```python
from build123d import *

# Parameters (mm, degrees)
BOSS_EXTRUDE1_DEPTH = 152.4
CUT_EXTRUDE1_DEPTH  = 1888.307171607
FILLET1_R           = 10
BOSS_EXTRUDE2_DEPTH = 476.835088
CUT_EXTRUDE2_REACH  = 1889.307
SKETCH4_W           = 50.8
SKETCH4_H           = 222.835087774
SKETCH6_R           = 15.875
CUT_EXTRUDE3_DEPTH  = 1677.259068793
SKETCH7_W           = 40
SKETCH7_H           = 102.835087774
SKETCH7_R           = 5
BOSS_EXTRUDE3_DEPTH = 25.4


with BuildPart() as part:
    # Sketch1 → Boss-Extrude1 (new body)
    with BuildSketch(Plane.XY):
        Polygon((0, 0), (-762, 0), (-1066.8, 304.8), (-1066.8, 787.4), (-812.8, 1549.4), (0, 1549.4), align=None)
    extrude(amount=BOSS_EXTRUDE1_DEPTH)

    # Sketch2 → Cut-Extrude1 (cut, through all)
    with BuildSketch(Plane.XY.offset(152.4)):
        Polygon((-924.463579053, 812.8), (-127, 939.8), (-127, 1435.1), (-717.03024572, 1435.1), align=None)
    extrude(amount=-CUT_EXTRUDE1_DEPTH, mode=Mode.SUBTRACT)

    # Fillet1
    fillet1_edges = [part.edges().sort_by_distance(p)[0] for p in [
        (0, 0, 76.2),
        (-762, 0, 76.2),
        (-1066.8, 304.8, 76.2),
        (-1066.8, 787.4, 76.2),
        (-812.8, 1549.4, 76.2),
        (0, 1549.4, 76.2),
        (-939.8, 1168.4, 152.4),
        (-1066.8, 546.1, 152.4),
        (-914.4, 152.4, 152.4),
        (-820.746912386, 1123.95, 0),
        (-924.463579053, 812.8, 76.2),
        (-422.01512286, 1435.1, 0),
        (-717.03024572, 1435.1, 76.2),
        (-127, 1187.45, 0),
        (-381, 0, 152.4),
        (-127, 1435.1, 76.2),
        (-525.731789526, 876.3, 0),
        (-127, 939.8, 76.2),
        (-820.746912386, 1123.95, 152.4),
        (-525.731789526, 876.3, 152.4),
        (-127, 1187.45, 152.4),
        (-422.01512286, 1435.1, 152.4),
        (0, 774.7, 152.4),
        (-381, 0, 0),
        (-914.4, 152.4, 0),
        (-1066.8, 546.1, 0),
        (-939.8, 1168.4, 0),
        (-406.4, 1549.4, 0),
        (0, 774.7, 0),
        (-406.4, 1549.4, 152.4),
    ]]
    fillet(fillet1_edges, radius=FILLET1_R)

    # Sketch3 → Boss-Extrude2 (add)
    with BuildSketch(Plane(origin=(0, 308.942135624, 0), x_dir=(-1, 0, 0), z_dir=(0, -1, 0))):
        with BuildLine():
            Line((1066.286832981, -76.2), (1066.286832981, -50.8))
            Line((1066.286832981, -50.8), (1091.686832981, -50.8))
            ThreePointArc((1091.686832981, -50.8), (1117.086832981, -76.2), (1091.686832981, -101.6))
            Line((1091.686832981, -101.6), (1066.286832981, -101.6))
            Line((1066.286832981, -101.6), (1066.286832981, -76.2))
        make_face()
    extrude(amount=-BOSS_EXTRUDE2_DEPTH)

    # Sketch4 → Cut-Extrude2 (cut, up to next)
    with BuildSketch(Plane.ZY.offset(1066.8), mode=Mode.PRIVATE) as cut_extrude2_sk1:
        with Locations((76.2, 547.359679511)):
            Rectangle(SKETCH4_W, SKETCH4_H)
    cut_extrude2_tool1 = extrude(cut_extrude2_sk1.sketch, amount=CUT_EXTRUDE2_REACH, mode=Mode.PRIVATE) & part.part
    add(cut_extrude2_tool1.solids().sort_by_distance((-1066.8, 547.35968, 76.2))[0], mode=Mode.SUBTRACT)

    # Sketch6 → Cut-Extrude3 (cut, through all)
    with BuildSketch(Plane(origin=(0, 308.942135624, 0), x_dir=(-1, 0, 0), z_dir=(0, -1, 0))):
        with Locations(Location((1091.686832981, -76.2, 0), (0, 0, 90))):
            Circle(SKETCH6_R)
    extrude(amount=-CUT_EXTRUDE3_DEPTH, mode=Mode.SUBTRACT)

    # Sketch7 → Boss-Extrude3 (add)
    with BuildSketch(Plane(origin=(0, 0, 0), x_dir=(-1, 0, 0), z_dir=(0, 0, -1))):
        with Locations((1036.8, 547.359679511)):
            Rectangle(SKETCH7_W, SKETCH7_H)
        with Locations((1036.8, 573.359679511)):
            Circle(SKETCH7_R, mode=Mode.SUBTRACT)
        with Locations((1036.8, 521.359679511)):
            Circle(SKETCH7_R, mode=Mode.SUBTRACT)
    extrude(amount=BOSS_EXTRUDE3_DEPTH)


solid = part.part
```
Verification items for the finished model (mm, model axes). A direction names the side the tool comes from. Coordinates: 2 decimals unless noted, no trailing zeros. Put each result on its own line as item: value. Start each with the question number.
1) Cross-section at A-A (z = 76.2). State how many separate pieces and enclosed holes the cut face has, plus the area to 3 significant figures.
2) Go/stop test with flat-tipped pins: pin 1 (2 mm diameter, centred on y = 1274.5, z = 111, fed in from -X); pin 2 (1 mm diameter, centred on y = 998.5, z = 79.5, fed in from -X); pin 3 (12.5 mm diameter, centred on y = 567, z = -15.5, fed in from -X). Record where each tip stops, or that it passes through.
3) Release check for a two-part mould opening along Z. For faces 1 (the cylindrical face through (-914.48, 156.51, 3.01)), 2 (the flat face through (-1066.8, 544, 75)), 3 (the cylindrical face through (-1107.184, 371.553, 79.641)), 4 (the cylindrical face through (-914.48, 156.51, 149.39)) record: pulls with the +Z half, pulls with the -Z half, needs draft (parallel to the pull), parting line crosses it, or undercut.
4) Tool access check on faces 5 (the cylindrical face through (-820.735, 1133.495, 2.852)), 6 (the flat face through (-127, 1183, 77)), 7 (the flat face through (-1075.5, 308.942, 75.8)), 8 (the flat face through (-1075, 435.942, 76)). Record the directions out of +Z, -Z, +X, -X, +Y, -Y that give a thin tool (end or side, any length) a straight path to the whole face; none if there is none.
5) Material ranges on L1, parallel to Y at x = -1036, z = -7; L2, parallel to Y at x = -1036.8, z = -14; L3, parallel to X at y = 377.5, z = 76.2, recorded low to high.
Geometry check:
1. separate pieces: 3
1. enclosed holes: 1
1. area: 1,130,000 mm^2
2. pin 1: stops at x = -904.77
2. pin 2: stops at x = -996.6
2. pin 3: stops at x = -1056.8
3. face 1: pulls with the -Z half
3. face 2: needs draft
3. face 3: undercut
3. face 4: pulls with the +Z half
4. face 5: -Z
4. face 6: +Z, -Z
4. face 7: +Z, -Z, -X, -Y
4. face 8: +Z, -Z, -X
5. L1: y = 495.94 to 516.42, 526.3 to 568.42, 578.3 to 598.78
5. L2: y = 495.94 to 516.36, 526.36 to 568.36, 578.36 to 598.78
5. L3: x = -1117.09 to -1107.56, -1075.81 to 0
